Autodesk Inventor part; units mm, degrees
ref_plane "YZ Plane" through (0, 0, 0) normal (1, 0, 0) x (0, 1, 0)
ref_plane "XZ Plane" through (0, 0, 0) normal (0, 1, 0) x (-1, 0, 0)
ref_plane "XY Plane" through (0, 0, 0) normal (0, 0, 1) x (1, 0, 0)
sketch "Boceto1" plane through (0, 0, 0) normal (1, 0, 0) x (0, 1, 0)
  circle A0 centre (0, 0) radius 65
  line L0 (0, 0) -> (-45.9619, 45.9619)
  line L1 (0, 0) -> (65, 0) construction
  line L2 (0, 0) -> (16.8232, -62.7852)
  line L3 (0, 0) -> (65, 0) construction
  circle A1 centre (0, 0) radius 15
  dimension "d5" = 130
  dimension "d6" = 135
  dimension "d7" = 75
  dimension "d8" = 30
extrude "Extrusión1" add sketch "Boceto1" along normal blind 10 contours A0 L2 A1 L0 | A1 L2 L0 | L0 L2 A1 picked at (40.3579, 26.2595)
sketch "Boceto2" plane through (0, 3.8823, -14.4889) normal (0, -0.9659258, -0.258819) x (1, 0, 0)
  line L0 (2, -20) -> (8, -20)
  line L1 (8, -20) -> (8, -48)
  line L2 (8, -48) -> (2, -48)
  line L3 (2, -48) -> (2, -20)
  line L4 (10, 0) -> (10, 27.9904)
  line L5 (0, -50) -> (10, -50)
  point P0 (0, 15)
  dimension "d11" = 6
  dimension "d12" = 28
  dimension "d18" = 2
revolve "Revolución1" cut sketch "Boceto2" angle 360 about axis through (2, 9.0587, -33.8074) along (1, 0, 0)
sketch "Boceto3" plane through (10, 0, 0) normal (1, 0, 0) x (0, 0, -1)
  circle A0 centre (0, 0) radius 10
  arc A1 (-10.6066, -10.6066) -> (14.4889, 3.8823) centre (0, 0) ccw
  dimension "d20" = 20
extrude "Extrusión2" cut sketch "Boceto3" against normal blind 10
sketch "Boceto4" plane through (0, 0, 0) normal (-1, 0, 0) x (0, 0, 1)
  point P0 (0, 0)
sketch "Boceto5" plane through (0, 0, 0) normal (-1, 0, 0) x (0, 0, 1)
  arc A0 (46.9928, -0.8201) -> (0, 47) centre (0, 0) ccw
  circle A1 centre (16.5227, 44) radius 4
  circle A2 centre (33.5227, 32.9428) radius 4
  dimension "d23" = 47
  dimension "d24" = 8
  dimension "d25" = 8
  dimension "d28" = 17
  dimension "d29" = 44
extrude "Extrusión3" cut sketch "Boceto5" against normal blind 2
properties part number "protector"
Design review of the part built by this model. Coordinates are the model's own, in mm. A direction names the side the tool comes from. Coordinates: 2 decimals unless noted, no trailing zeros. Write each loop counter-clockwise with the first axis right and the second up, starting at its lowest first coordinate (ties: lowest second). Pieces come first, ordered by that corner, then holes.
1) Add section B-B (z = 0). Write out the cut boundary in (x, y).
2) Add section C-C (z = -38.5). Write out the cut boundary in (x, y).
3) To check wall thickness, follow L1, parallel to X at y = 5, z = -13; L2, parallel to Y at x = 3.25, z = 0; L3, parallel to Z at x = 0.5, y = 44. State the ranges of each line that lie inside material, in increasing order.
4) Machinability: for faces 4 (the cylindrical face through (4.958, -6.543, -10.557)), 5 (the flat face through (2, 21, -30)), 6 (the flat face through (2, 33, 33)), which of the approach directions +Z, -Z, +X, -X, +Y, -Y give a long, thin tool a straight path to every point of the face, cutting with its end or side? Answer none if there is none.
5) Add section D-D (x = 4). Write out the cut boundary in (y, z).
6) Add section A-A (y = 0). Write out the cut boundary in (x, z), plus the area to 3 significant figures.
7) Mouldability with a two-part tool opening along Z and no side actions: class faces 1 (the flat face through (0, 21, 16)), 2 (the flat face through (1.597, 10.262, -38.299)), 3 (the flat face through (8, 21, -30)) as +Z half, -Z half, draft (parallel to the pull), parting line (faces both ways), or undercut.
8) Insertion check: pin 1 (13 mm diameter, centred on y = 44, z = 16.52, fed in from -X); pin 2 (3 mm diameter, centred on x = 7.5, y = 14, fed in from +Z); pin 3 (2 mm diameter, centred on x = 6, y = -29.5, fed in from -Z); pin 4 (2.5 mm diameter, centred on y = 31, z = 33, fed in from -X). Each pin has a flat end and moves straight along its axis. Give the tip position at first contact, or say it passes through.
Check result:
1. outline: (0, -15) - (10, -15) - (10, -10) - (0, -10) - close; (0, 10) - (10, 10) - (10, 65) - (0, 65) - close
2. outline: (0, 10.32) - (2, 10.32) - (2, 36.66) - (8, 36.66) - (8, 10.32) - (10, 10.32) - (10, 52.37) - (0, 52.37) - close
3. L1: x = 0 to 2, 8 to 10
3. L2: y = -15 to -10, 10 to 65
3. L3: z = -47.84 to 12.52, 20.52 to 47.84
4. face 4: -Z
4. face 5: none
4. face 6: -X
5. outline: (-45.96, 45.96) - (-10.61, 10.61) arc R15 ccw to (-8.74, -12.19) arc R28 cw to (-4.13, -9.11) arc R10 cw (long way) to (8.13, -5.82) arc R28 cw to (16.31, -60.85) - (16.82, -62.79) arc R65 ccw (long way) to start
6. outline: (0, -15) - (2, -15) - (2, -10) - (0, -10) - close; (0, 10) - (10, 10) - (10, 65) - (0, 65) - close; (8, -15) - (10, -15) - (10, -10) - (8, -10) - close
6. area: 570 mm2
7. face 1: draft
7. face 2: -Z half
7. face 3: undercut
8. pin 1: stops at x = 0
8. pin 2: stops at z = 63.79
8. pin 3: stops at z = 28.5
8. pin 4: stops at x = 2
